The model under review builds one solid part; all positions refer to its coordinate system, in mm. A direction names the side the tool comes from. Give positions to 0.01 mm unless a question says otherwise; leave off trailing zeros. Loops run counter-clockwise (first coordinate to the right, second up) from the corner with the lowest first, then second, coordinate; pieces in that order, holes last. Notation, with made-up numbers: M 54.5,74 L 107.5,74 A29 cw 107.5,94 Z; hole C -25.5,-20.75 d8. An arc over 180 degrees is marked long. Return JSON: item names as keys, results as strings.
```python
from build123d import *

# Parameters (mm, degrees)
SKETCH_W     = 48.4
SKETCH_H     = 25.7
PAD_DEPTH    = 5
SKETCH001_W  = 8
SKETCH001_H  = 3
PAD001_DEPTH = 1.5
SKETCH002_R  = 1.65
POCKET_DEPTH = 5.001


with BuildPart() as part:
    # Sketch → Pad (new body)
    with BuildSketch(Plane.XY):
        Rectangle(SKETCH_W, SKETCH_H)
    extrude(amount=PAD_DEPTH)

    # Sketch001 (on Face4 of Pad) → Pad001 (join)
    with BuildSketch(Plane(origin=(-24.2, 0, 0), x_dir=(0, -1, 0), z_dir=(-1, 0, 0))):
        with Locations((0, 3.5)):
            Rectangle(SKETCH001_W, SKETCH001_H)
    extrude(amount=PAD001_DEPTH)

    # Sketch002 (on Face5 of Pad001) → Pocket (cut, through all)
    with BuildSketch(Plane.XY.offset(5)):
        with Locations((-21, 10.5)):
            Circle(SKETCH002_R)
        with Locations((-21, -10.5)):
            Circle(SKETCH002_R)
        with Locations((21, 10.5)):
            Circle(SKETCH002_R)
        with Locations((21, -10.5)):
            Circle(SKETCH002_R)
    extrude(amount=-POCKET_DEPTH, mode=Mode.SUBTRACT)


with BuildPart() as part_1:
    # Body placement: moved
    add(part.part.moved(Location((0, 0, 6.5))))


solid = part_1.part
```
1) Insertion check: pin 1 (2 mm diameter, centred on x = 21, y = -10.5, fed in from -Z); pin 2 (1.2 mm diameter, centred on x = -25, z = 10.5, fed in from +Y). Each pin has a flat end and moves straight along its axis. Give the tip position at first contact, or say it passes through.
From the geometry:
{"pin 1": "through", "pin 2": "y = 4"}
2) Wall thickness on L1, parallel to Y at x = -21, z = 8.95; L2, parallel to X at y = -9.25, z = 10.7; L3, parallel to X at y = -9.75, z = 9.9: over which ranges is each line inside the solid? List them lowest first. Write a range as from..to.
From the geometry:
{"L1": "-12.85..-12.15, -8.85..8.85, 12.15..12.85", "L2": "-24.2..-22.08, -19.92..19.92, 22.08..24.2", "L3": "-24.2..-22.47, -19.53..19.53, 22.47..24.2"}
3) The part is to be moulded in two halves that separate along X. For faces 1 (the face through (-25, 0, 8.5)), 2 (the face through (-22.31, 9.5, 9.04)), 3 (the face through (-25.7, 0, 10)), 4 (the face through (24.2, 0, 9)), say which applies: released by +X, released by -X, zero draft, split by the parting line, or undercut.
From the geometry:
{"face 1": "zero draft", "face 2": "undercut", "face 3": "released by -X", "face 4": "released by +X"}
4) Consider section D-D on z = 10.45. Write out the cut boundary in (x, y).
From the geometry:
{"outline": "M -25.7,-4 L -24.2,-4 L -24.2,-12.85 L 24.2,-12.85 L 24.2,12.85 L -24.2,12.85 L -24.2,4 L -25.7,4 Z; hole C -21,-10.5 d3.3; hole C -21,10.5 d3.3; hole C 21,-10.5 d3.3; hole C 21,10.5 d3.3"}
5) Tool access review of faces 5 (the face through (0, -12.85, 9)), 6 (the face through (-25, 4, 10)), 7 (the face through (-25, -4, 10)): name each direction out of +Z, -Z, +X, -X, +Y, -Y from which nothing blocks a thin tool from reaching the whole face with its end or side.
From the geometry:
{"face 5": "+Z, -Z, +X, -X, -Y", "face 6": "+Z, -Z, -X, +Y", "face 7": "+Z, -Z, -X, -Y"}
6) Consider section C-C on z = 7.7. Write out the cut boundary in (x, y).
From the geometry:
{"outline": "M -24.2,-12.85 L 24.2,-12.85 L 24.2,12.85 L -24.2,12.85 Z; hole C -21,-10.5 d3.3; hole C -21,10.5 d3.3; hole C 21,-10.5 d3.3; hole C 21,10.5 d3.3"}
7) Consider section B-B on x = -21. Write out the cut boundary in (y, z), then the cut area to 3 significant figures.
From the geometry:
{"outline": "M -12.85,6.5 L -12.15,6.5 L -12.15,11.5 L -12.85,11.5 Z; M -8.85,6.5 L 8.85,6.5 L 8.85,11.5 L -8.85,11.5 Z; M 12.15,6.5 L 12.85,6.5 L 12.85,11.5 L 12.15,11.5 Z", "area": "95.5 mm²"}
8) Consider section A-A on y = 10.5. Write out the cut boundary in (x, z).
From the geometry:
{"outline": "M -24.2,6.5 L -22.65,6.5 L -22.65,11.5 L -24.2,11.5 Z; M -19.35,6.5 L 19.35,6.5 L 19.35,11.5 L -19.35,11.5 Z; M 22.65,6.5 L 24.2,6.5 L 24.2,11.5 L 22.65,11.5 Z"}
